Geometry: final body of the model. Coordinates: model frame, mm. Face numbers are marked on the shaded views. A direction names the side the tool comes from. Round coordinates to 2 decimals unless told otherwise and drop trailing zeros. Loops run counter-clockwise (first coordinate to the right, second up) from the corner with the lowest first, then second, coordinate; pieces in that order, holes last. Notation, with made-up numbers: (5.5, 80.5) -> (28.5, 80.5) arc R31 ccw to (28.5, 108.5) -> close; hole circle Ø2 at (84, 77.5). An arc over 180 degrees is marked (long way). Answer in a Markdown table with one row per item.
```python
from build123d import *

# Parameters (mm, degrees)
SKETCH1_W               = 31
SKETCH1_H               = 21
BOSS_EXTRUDE1_DEPTH     = 15
M2_CLEARANCE_HOLE1_D    = 2.2
SKETCH10_R              = 10.5
BOSS_EXTRUDE3_DEPTH     = 3
SKETCH7_R               = 1.25
SKETCH7_R_2             = 2.5
CUT_EXTRUDE1_DEPTH      = 4
CUT_EXTRUDE1_DEPTH_BACK = 16


with BuildPart() as part:
    # Sketch1 → Boss-Extrude1 (new body)
    with BuildSketch(Plane(origin=(0, 0, 0), x_dir=(0, 0, -1), z_dir=(1, 0, 0))):
        Rectangle(SKETCH1_W, SKETCH1_H)
    extrude(amount=BOSS_EXTRUDE1_DEPTH)

    # M2 Clearance Hole1 (through all)
    with Locations(Plane.XY.offset(15.5)):
        with Locations((2, 0)):
            Hole(M2_CLEARANCE_HOLE1_D / 2)

    # Sketch10 → Boss-Extrude3 (add)
    with BuildSketch(Plane(origin=(15, 0, 0), x_dir=(0, 0, -1), z_dir=(1, 0, 0))):
        Circle(SKETCH10_R)
    extrude(amount=BOSS_EXTRUDE3_DEPTH)

    # Sketch7 → Cut-Extrude1 (cut, two sides)
    with BuildSketch(Plane(origin=(15, 0, 0), x_dir=(0, 0, -1), z_dir=(1, 0, 0))) as cut_extrude1_sk:
        with Locations((-5, 0)):
            Circle(SKETCH7_R)
        with Locations((5, 0)):
            Circle(SKETCH7_R)
        Circle(SKETCH7_R_2)
    extrude(amount=CUT_EXTRUDE1_DEPTH, mode=Mode.SUBTRACT)
    extrude(cut_extrude1_sk.sketch, amount=-CUT_EXTRUDE1_DEPTH_BACK, mode=Mode.SUBTRACT)


solid = part.part
```
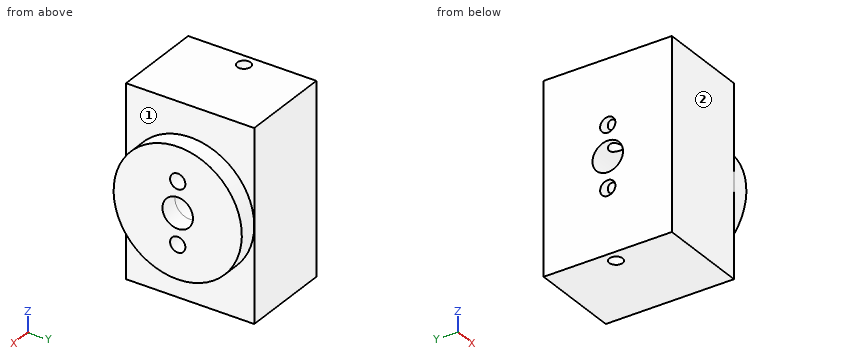
Item 1: Set-up query: the marked faces 1 and 2. Return all of +Z, -Z, +X, -X, +Y, -Y with unobstructed straight access to the full face (end or side cutting, diameter ignored); none if empty.
Ans:
| item | result |
|---|---|
| face 1 | +Z, +X |
| face 2 | +Z, -Z, +X, -X, -Y |
Item 2: Section query C-C, the plane y = 0. State how many separate pieces and enclosed holes the cut face has, and give its area (3 significant figures).
Ans:
| item | result |
|---|---|
| separate pieces | 8 |
| enclosed holes | 0 |
| area | 302 mm2 |
Item 3: Section query D-D, the plane x = 12.75. Output: boundary loops of the cut face in (y, z), and give its area (3 significant figures).
Ans:
| item | result |
|---|---|
| outline | (-10.5, -15.5) -> (10.5, -15.5) -> (10.5, 15.5) -> (-10.5, 15.5) -> close; hole circle Ø5 at (0, 0); hole circle Ø2.5 at (0, -5); hole circle Ø2.5 at (0, 5) |
| area | 622 mm2 |
Item 4: Section query B-B, the plane z = 5. Output: boundary loops of the cut face in (x, y).
Ans:
| item | result |
|---|---|
| outline | (0, -10.5) -> (15, -10.5) -> (15, -9.23) -> (18, -9.23) -> (18, -1.25) -> (0, -1.25) -> close; (0, 1.25) -> (18, 1.25) -> (18, 9.23) -> (15, 9.23) -> (15, 10.5) -> (0, 10.5) -> close |
Item 5: Ray query, L1, parallel to Z at x = 16.1, y = 0; L2, parallel to Z at x = 6, y = 0; L3, parallel to Y at x = 2, z = 9. Return the intervals inside material, ascending.
Ans:
| item | result |
|---|---|
| L1 | -10.5 to -6.25, -3.75 to -2.5, 2.5 to 3.75, 6.25 to 10.5 |
| L2 | -15.5 to -6.25, -3.75 to -2.5, 2.5 to 3.75, 6.25 to 15.5 |
| L3 | -10.5 to -1.1, 1.1 to 10.5 |
Item 6: Section query A-A, the plane x = 2. Output: boundary loops of the cut face in (y, z) (3 decimals).
Ans:
| item | result |
|---|---|
| outline | (-10.5, -15.5) -> (-1.1, -15.5) -> (-1.1, -5.594) arc R1.25 cw to (-1.1, -4.406) -> (-1.1, -2.245) arc R2.5 cw to (-1.1, 2.245) -> (-1.1, 4.406) arc R1.25 cw to (-1.1, 5.594) -> (-1.1, 15.5) -> (-10.5, 15.5) -> close; (1.1, -15.5) -> (10.5, -15.5) -> (10.5, 15.5) -> (1.1, 15.5) -> (1.1, 5.594) arc R1.25 cw to (1.1, 4.406) -> (1.1, 2.245) arc R2.5 cw to (1.1, -2.245) -> (1.1, -4.406) arc R1.25 cw to (1.1, -5.594) -> close |
